Design review of the part shown in the three views and the two pictorial views. Dimensions are in mm from the part's minimum x, y and z. Round coordinates to 2 decimals unless told otherwise and drop trailing zeros. Loops run counter-clockwise (first coordinate to the right, second up) from the corner with the lowest first, then second, coordinate; pieces in that order, holes last.
1. Consider section B-B on z = 28. State the section outline as (x, y) points, then the cut area to 3 significant figures.
2. Draft analysis for pull direction Z (two halves, no side actions). For the marked faces 1, 2 and 3, state which applies: released by +Z, released by -Z, zero draft, split by the parting line, or undercut.
3. Consider section C-C on x = 20. State the section outline as (y, z) points.
4. To check wall thickness, follow line 1 along Z through (x, y) = (20, 5.3); line 2 along X through (y, z) = (4.8, 12). State the ranges of each line that lie inside material, in increasing order.
5. Clearance check with a flat-ended pin moving along its axis: pin 1 Ø4 at (x, z) = (28, 20) entering from -Y. State where the tip first meets the part, or that it passes through.
6. Consider section A-A on x = 12. State the section outline as (y, z) points, then the cut area to 3 significant figures.
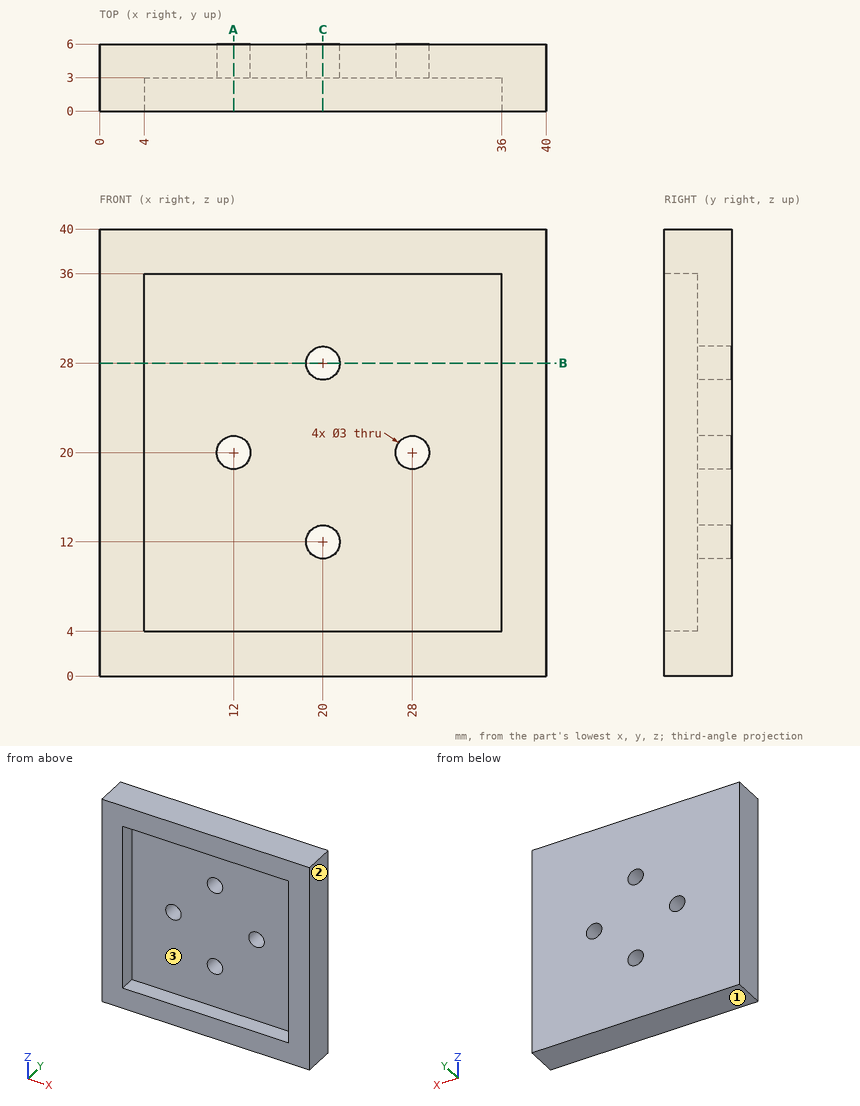
Resolved:
1. outline: (0, 0) - (4, 0) - (4, 3) - (18.5, 3) - (18.5, 6) - (0, 6) - close; (21.5, 3) - (36, 3) - (36, 0) - (40, 0) - (40, 6) - (21.5, 6) - close
1. area: 135 mm2
2. face 1: released by -Z
2. face 2: zero draft
2. face 3: undercut
3. outline: (0, 0) - (6, 0) - (6, 10.5) - (3, 10.5) - (3, 4) - (0, 4) - close; (0, 36) - (3, 36) - (3, 29.5) - (6, 29.5) - (6, 40) - (0, 40) - close; (3, 13.5) - (6, 13.5) - (6, 26.5) - (3, 26.5) - close
4. line 1: z = 0 to 10.5, 13.5 to 26.5, 29.5 to 40
4. line 2: x = 0 to 18.5, 21.5 to 40
5. pin 1: stops at y = 3
6. outline: (0, 0) - (6, 0) - (6, 18.5) - (3, 18.5) - (3, 4) - (0, 4) - close; (0, 36) - (3, 36) - (3, 21.5) - (6, 21.5) - (6, 40) - (0, 40) - close
6. area: 135 mm2
